Model file for the job. Use its own axes, mm. Round coordinates to 2 decimals unless told otherwise and drop trailing zeros. Order: outer loops, then holes, each group sorted by start corner. A loop starts at its lowest first (then second) coordinate and runs counter-clockwise, first axis right, second up. Notation, with made-up numbers: (70, 78) -> (95, 78) arc R23 ccw to (95, 90) -> close; hole circle Ø2 at (-29, 46.25). An arc over 180 degrees is marked (long way). Answer as CSV lines item,"result".
```python
from build123d import *

# Parameters (mm, degrees)
F0_W     = 60
F0_H     = 20.115981
F0_R     = 3
F0_R_2   = 1.308767
F1_DEPTH = 10
F3_R     = 6


with BuildPart() as f1:
    # F0 (on Front) → F1 (new body)
    with BuildSketch(Plane.XZ):
        with Locations((30, 10.05799)):
            Rectangle(F0_W, F0_H)
        with Locations((6.314433, 11.456186)):
            Circle(F0_R, mode=Mode.SUBTRACT)
        with Locations((26.120204, 12.682377)):
            Circle(F0_R_2, mode=Mode.SUBTRACT)
        with Locations((50, 11.406668)):
            Circle(F0_R, mode=Mode.SUBTRACT)
    extrude(amount=F1_DEPTH)

    # F3
    f3_edges = [f1.edges().sort_by_distance(p)[0] for p in [
        (0, -5, 0),
        (0, -5, 20.115981),
        (60, -5, 0),
        (60, -5, 20.115981),
    ]]
    fillet(f3_edges, radius=F3_R)


solid = f1.part
```
Q1. Saw through at A-A (x = 50). Write the cut outline in (y, z), plus the area to 3 significant figures.
Checks:
outline,"(-10, 0) -> (0, 0) -> (0, 8.41) -> (-10, 8.41) -> close; (-10, 14.41) -> (0, 14.41) -> (0, 20.12) -> (-10, 20.12) -> close"
area,"141 mm²"
Q2. Saw through at B-B (y = -6.5). Write the cut outline in (x, z), plus the area to 3 significant figures.
Checks:
outline,"(0, 6) arc R6 ccw to (6, 0) -> (54, 0) arc R6 ccw to (60, 6) -> (60, 14.12) arc R6 ccw to (54, 20.12) -> (6, 20.12) arc R6 ccw to (0, 14.12) -> close; hole circle Ø6 at (6.31, 11.46); hole circle Ø2.62 at (26.12, 12.68); hole circle Ø6 at (50, 11.41)"
area,"1,110 mm²"
Q3. Mould opens along X. For faces 1 (the cylindrical face through (27.369, -4.93, 13.075)), 2 (the flat face through (30, -5, 0)), 3 (the cylindrical face through (1.711, -5.07, 1.804)), 4 (the cylindrical face through (58.196, -5.07, 1.711)) say: +X half, -X half, draft (parallel to the pull), parting line (faces both ways), or undercut.
Checks:
face 1,"undercut"
face 2,"draft"
face 3,"-X half"
face 4,"+X half"
Q4. Saw through at C-C (z = 2.75). Write the cut outline in (x, y).
Checks:
outline,"(0.96, -10) -> (59.04, -10) -> (59.04, 0) -> (0.96, 0) -> close"
Q5. Wall check: L1, parallel to Z at x = 50, y = -7.5; L2, parallel to X at y = -5, z = 8.75; L3, parallel to X at y = -1, z = 12.5. Give the ranges that are in metal, low to high. Write a range as [from, to].
Checks:
L1,"[0, 8.41], [14.41, 20.12]"
L2,"[0, 5.02], [7.61, 48.61], [51.39, 60]"
L3,"[0, 3.5], [9.13, 24.82], [27.42, 47.21], [52.79, 60]"
